Study the drawing (mm; zero at the part's minimum x, y, z) and answer. A direction names the side the tool comes from. Round coordinates to 2 decimals unless told otherwise and drop trailing zeros. Write each loop counter-clockwise with the first axis right and the second up, starting at its lowest first coordinate (ties: lowest second). Pieces come first, ordered by that corner, then holes. Notation, with made-up numbers: M 32,36.5 L 48,36.5 A12 ccw 48,48.5 Z; hole C 28.25,34 d6. An arc over 180 degrees is marked long. Write each question's results on one line, items separated by ' | '.
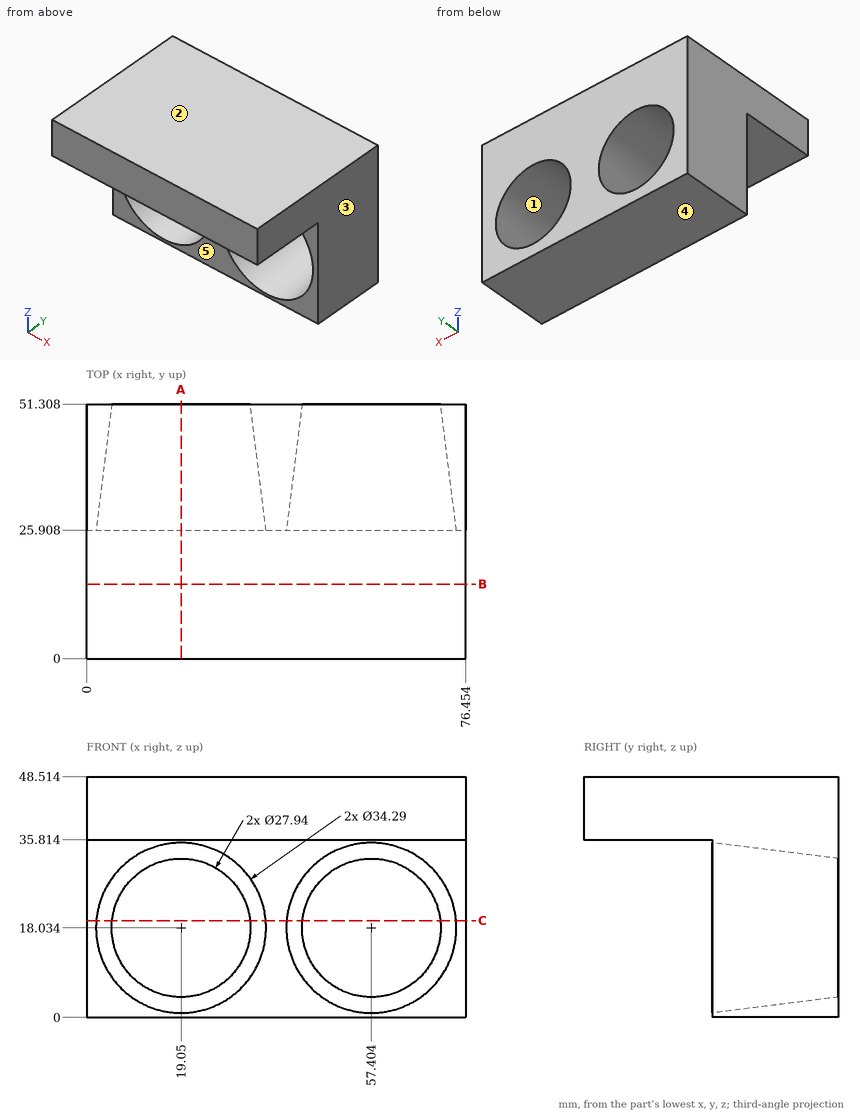
1) Section B-B (y = 15) is taken. Determine the outline of the cut face in (x, z).
Return value:
outline: M 0,35.81 L 76.45,35.81 L 76.45,48.51 L 0,48.51 Z
2) This flat-tipped pin is pushed along its axis until it touches: pin 1 (13 mm diameter, centred on x = 43.5, y = 18, fed in from -Z). Where does it stop, or does it pass through?
Return value:
pin 1: z = 35.81
3) Section C-C (z = 19.5) is taken. State how many separate pieces and enclosed holes the cut face has, then the cut area to 3 significant figures.
Return value:
separate pieces: 3 | enclosed holes: 0 | area: 368 mm²
4) Section A-A (x = 19.05) is taken. Determine the outline of the cut face in (y, z), then the cut area to 3 significant figures.
Return value:
outline: M 0,35.81 L 25.91,35.81 L 25.91,35.18 L 51.31,32 L 51.31,48.51 L 0,48.51 Z; M 25.91,0 L 51.31,0 L 51.31,4.06 L 25.91,0.89 Z | area: 771 mm²
5) A tool of negligible diameter and unlimited length cuts with its end or side. For the marked faces 4 and 5, from which of +Z, -Z, +X, -X, +Y, -Y can it reach the whole face along a straight path? Write none if from no direction.
Return value:
face 4: -Z, +X, -X, +Y, -Y | face 5: -Z, +X, -X, -Y
6) The mould has two halves that part along X. Classify the marked faces 1, 2 and 3: +X half, -X half, draft (parallel to the pull), parting line (faces both ways), or undercut.
Return value:
face 1: undercut | face 2: draft | face 3: +X half
7) Find the intervals of material crossed by line 1 (X direction, y = 41.5, z = 14.5); line 2 (X direction, y = 37.5, z = 31.5); line 3 (Z direction, x = 35.5, y = 17), in increasing order.
Return value:
line 1: 0 to 4.27, 33.83 to 42.62, 72.18 to 76.45 | line 2: 0 to 10.99, 27.11 to 49.34, 65.47 to 76.45 | line 3: 35.81 to 48.51
